```python
from build123d import *

# Parameters (mm, degrees)
CUT_EXTRUDE1_DEPTH      = 41
CUT_EXTRUDE1_DEPTH_BACK = 20
SKETCH1_5_R             = 1.05
CUT_EXTRUDE2_DEPTH      = 20
CUT_EXTRUDE2_DEPTH_BACK = 20
SKETCH1_6_R             = 1.05
CHAMFER1_SIZE           = 2.5
CHAMFER2_SIZE           = 2.5


with BuildPart() as part:
    # Sketch1 → Revolve1 (revolve)
    with BuildSketch(Plane.XY, mode=Mode.PRIVATE) as revolve1_sk:
        with BuildLine():
            ThreePointArc((34.95, 0), (36, 1.05), (37.05, 0))
            Line((37.05, 0), (48, 0))
            Line((48, 0), (48, 5))
            Line((48, 5), (-48, 5))
            Line((-48, 5), (-48, 0))
            Line((-48, 0), (-37.05, 0))
            ThreePointArc((-37.05, 0), (-36, 1.05), (-34.95, 0))
            Line((-34.95, 0), (34.95, 0))
        make_face()
        with BuildLine():
            ThreePointArc((-37.05, 0), (-36, -1.05), (-34.95, 0))
            Line((-34.95, 0), (-37.05, 0))
        make_face()
        with BuildLine():
            Line((-37.05, 0), (-34.95, 0))
            ThreePointArc((-34.95, 0), (-36, 1.05), (-37.05, 0))
        make_face()
        with BuildLine():
            ThreePointArc((34.95, 0), (36, -1.05), (37.05, 0))
            Line((37.05, 0), (34.95, 0))
        make_face()
        with BuildLine():
            Line((34.95, 0), (37.05, 0))
            ThreePointArc((37.05, 0), (36, 1.05), (34.95, 0))
        make_face()
    revolve(revolve1_sk.sketch.rotate(Axis((-48, 0, 0), (1, 0, 0)), 180), axis=Axis((-48, 0, 0), (1, 0, 0)))

    # Sketch1_5 → Cut-Extrude1 (cut, two sides: drawn at the far end of the back side and taken through both)
    with BuildSketch(Plane.XY.offset(-CUT_EXTRUDE1_DEPTH_BACK)):
        with Locations(Location((-36, 0, 0), (0, 0, 180))):
            Circle(SKETCH1_5_R)
    extrude(amount=CUT_EXTRUDE1_DEPTH + CUT_EXTRUDE1_DEPTH_BACK, mode=Mode.SUBTRACT)

    # Sketch1_6 → Cut-Extrude2 (cut, two sides: drawn at the far end of the back side and taken through both)
    with BuildSketch(Plane.XY.offset(-CUT_EXTRUDE2_DEPTH_BACK)):
        with Locations(Location((36, 0, 0), (0, 0, 180))):
            Circle(SKETCH1_6_R)
    extrude(amount=CUT_EXTRUDE2_DEPTH + CUT_EXTRUDE2_DEPTH_BACK, mode=Mode.SUBTRACT)

    # Chamfer1
    chamfer1_edges = [part.edges().sort_by_distance(p)[0] for p in [
        (-48, 5, 0),
    ]]
    chamfer(chamfer1_edges, length=CHAMFER1_SIZE)

    # Chamfer2
    chamfer2_edges = [part.edges().sort_by_distance(p)[0] for p in [
        (48, 5, 0),
    ]]
    chamfer(chamfer2_edges, length=CHAMFER2_SIZE)


solid = part.part
```
Work out the finished part from the listing and answer in its coordinate system (mm). Coordinates: 2 decimals unless noted, no trailing zeros. Loops run counter-clockwise (first coordinate to the right, second up) from the corner with the lowest first, then second, coordinate; pieces in that order, holes last.
1) Section D-D (x = -36) is taken. Give the vertices of the cut face in (y, z).
Results:
outline: (-1.05, -4.89) - (-1.05, 4.89) arc R5 ccw to start; (1.05, -4.89) arc R5 ccw to (1.05, 4.89) - close
2) Section B-B (z = 0) is taken. Give the vertices of the cut face in (x, y), plus the area to 3 significant figures.
Results:
outline: (-48, -2.5) - (-45.5, -5) - (45.5, -5) - (48, -2.5) - (48, 2.5) - (45.5, 5) - (-45.5, 5) - (-48, 2.5) - close; hole circle Ø2.1 at (-36, 0); hole circle Ø2.1 at (36, 0)
area: 941 mm2
3) For a pull along Y with two mould halves and no side action, classify faces 1 (the cylindrical face through (-1, 5, 0)), 2 (the flat face through (48, 0, 0)), 3 (the cylindrical face through (37.05, -0.05, -0.07)) as +Y half, -Y half, draft (parallel to the pull), parting line (faces both ways), or undercut.
Results:
face 1: parting line
face 2: draft
face 3: undercut
4) Section A-A (y = 0) is taken. Give the vertices of the cut face in (x, z), plus the area to 4 significant figures.
Results:
outline: (-48, -2.5) - (-45.5, -5) - (-37.05, -5) - (-37.05, 5) - (-45.5, 5) - (-48, 2.5) - close; (-34.95, -5) - (34.95, -5) - (34.95, 5) - (-34.95, 5) - close; (37.05, -5) - (45.5, -5) - (48, -2.5) - (48, 2.5) - (45.5, 5) - (37.05, 5) - close
area: 905.5 mm2
5) Consider probe 1 along X at (y, z) = (-0.25, -3.25); probe 2 along Y at (x, z) = (-36, 2); probe 3 along Y at (x, z) = (36, 2.75). Determine where each line is inside the solid, lowest interval first.
Results:
probe 1: x = -47.24 to -37.02, -34.98 to 34.98, 37.02 to 47.24
probe 2: y = -4.58 to -1.05, 1.05 to 4.58
probe 3: y = -4.18 to -1.05, 1.05 to 4.18
6) Flat-ended cylindrical pins translate along their axes: pin 1 (1 mm diameter, centred on x = -27.5, y = 3.5, fed in from +Z); pin 2 (2 mm diameter, centred on x = -33, y = -2.5, fed in from +Z). Find the tip coordinate at first contact, or state that the pin passes through.
Results:
pin 1: stops at z = 4
pin 2: stops at z = 4.77
7) Section C-C (x = 27) is taken. Give the vertices of the cut face in (y, z).
Results:
outline: circle Ø10 at (0, 0)
